Source: CAD feature listing. Evaluate the final solid. Frame: model axes, mm. Face numbers are marked on the shaded views. A direction names the side the tool comes from. Give positions to 0.01 mm unless a question says otherwise; leave off trailing zeros. Order: outer loops, then holes, each group sorted by start corner. A loop starts at its lowest first (then second) coordinate and runs counter-clockwise, first axis right, second up. Notation, with made-up numbers: M 70,80 L 81,80 A29 cw 81,117 Z; hole C 57.25,1 d8. An arc over 180 degrees is marked long. Return JSON: item names as keys, results as strings.
Autodesk Inventor part; units mm, degrees
ref_plane "YZ Plane" through (0, 0, 0) normal (1, 0, 0) x (0, 1, 0)
ref_plane "XZ Plane" through (0, 0, 0) normal (0, 1, 0) x (-1, 0, 0)
ref_plane "XY Plane" through (0, 0, 0) normal (0, 0, 1) x (1, 0, 0)
sketch "スケッチ1" plane through (0, 0, 0) normal (0, 1, 0) x (-1, 0, 0)
  circle A0 centre (0, 0) radius 1.15
  circle A1 centre (0, 0) radius 2
  circle A2 centre (0, 0) radius 3
  line L0 (0, 0) -> (0, 3)
  line L1 (-2, 0) -> (2, 0)
  line L2 (2, 0) -> (2, -3)
  line L3 (2, -3) -> (-2, -3)
  line L4 (-2, -3) -> (-2, 0)
  line L5 (0, 0) -> (3, 0)
  line L6 (3, 0) -> (3, 3)
  line L7 (3, 3) -> (0, 3)
  line L8 (0, 3) -> (0, 0)
  point P0 (-2, -2.2361)
  point P1 (0, 2)
  point P2 (2, -2.2361)
  dimension "d1" = 4
  dimension "d2" = 6
  dimension "d0" = 2.3
extrude "押し出し1" add sketch "スケッチ1" along normal blind 3.2 contours A1 L4 A2 L0
extrude "押し出し2" add sketch "スケッチ1" along normal blind 4.5 contours L5 A2 L2 | A1 L0 A2 L5 | A2 L7 L6
extrude "押し出し3" add sketch "スケッチ1" against normal blind 1 contours L1 A1 A0 | A0 L0 A1 L1 | A0 L1 A1 L0 | L2 A2 L4 A1 | L5 A2 L2 | A1 L0 A2 L5 | A1 L4 A2 L0 | A2 L7 L6
sketch "スケッチ2" plane through (0, 4.5, 0) normal (0, 1, 0) x (1, 0, 0)
  circle A0 centre (0, 0) radius 1.15
  circle A1 centre (0, 0) radius 2
  circle A2 centre (0, 0) radius 3
  line L0 (0, 0) -> (-3, 0)
  line L1 (-3, 0) -> (-3, -3)
  line L2 (-3, -3) -> (0, -3)
  line L3 (0, -3) -> (0, 0)
  dimension "d9" = 2.3
  dimension "d10" = 4
  dimension "d11" = 6
extrude "押し出し4" add sketch "スケッチ2" along normal blind 1 contours A0 L0 A1 L3 | A0 L3 A1 L0 | L0 A2 L3 A1 | A1 L3 A2 L0 | A2 L2 L1
sketch "スケッチ3" plane through (-3, -1, 3) normal (0, 0, 1) x (1, 0, 0)
  line L0 (0, 6.5) -> (0, 0)
  line L1 (3, 5.5) -> (3, 6.5)
  line L2 (0, 0) -> (3, 0)
  line L3 (3, 0) -> (3, 6.5)
  line L4 (3, 6.5) -> (0, 6.5)
  line L5 (0, 6.5) -> (0, 0)
  point P0 (3, 1)
extrude "押し出し5" add sketch "スケッチ3" along normal blind 7
sketch "スケッチ4" plane through (-3, -1, 10) normal (0, 0, 1) x (1, 0, 0)
  line L0 (4.15, 0) -> (1.85, 0)
  line L1 (3, 0) -> (1.5, 0)
  line L2 (1.5, 0) -> (1.5, 1.5)
  line L3 (1.5, 1.5) -> (3, 1.5)
  line L4 (3, 1.5) -> (3, 0)
  point P0 (3, 1)
  dimension "d16" = 1.5
  dimension "d17" = 1.5
hole "穴1" at (-1.5, 0.5, 10) direction (0, 0, -1) diameter 1 end through all
sketch "スケッチ5" plane through (0, 3.2, 3) normal (1, 0, 0) x (0, 0, -1)
  point P0 (3, -3.2)
sketch "スケッチ7" plane through (0, 5.5, 0) normal (0, 1, 0) x (1, 0, 0)
  line L0 (0, -3) -> (0, -10)
  line L1 (0, -10) -> (-3, -10)
  line L2 (-3, -10) -> (-3, -50)
  line L3 (-3, -50) -> (0, -50)
  line L4 (0, -50) -> (0, -10)
  point P0 (0, 0)
  dimension "d33" = 3
  dimension "d34" = 40
sketch "スケッチ8" plane through (-3, -1, 10) normal (0, 0, 1) x (1, 0, 0)
  line L0 (0, 0) -> (0, 6.5)
  line L1 (0, 6.5) -> (4, 6.5)
  line L2 (4, 6.5) -> (4, 2.5)
  line L3 (4, 2.5) -> (0, 2.5)
  line L4 (0, 2.5) -> (0, 6.5)
  point P0 (3, 1)
  dimension "d35" = 4
  dimension "d36" = 4
extrude "押し出し7" add sketch "スケッチ8" along normal mid plane 8
sketch "スケッチ9" plane through (-3, -1, 14) normal (0, 0, 1) x (1, 0, 0)
  line L0 (0, 0) -> (0, 6.5)
  line L1 (0, 6.5) -> (2, 6.5)
  line L2 (2, 6.5) -> (2, 4.5)
  line L3 (2, 4.5) -> (0, 4.5)
  line L4 (0, 4.5) -> (0, 6.5)
  point P0 (3, 1)
  dimension "d39" = 2
  dimension "d40" = 2
hole "穴2" at (-1, 3.5, 14) direction (0, 0, -1) diameter 2 depth 3 tip angle 118
fillet "フィレット1" radius 2 1 edges at (1, 3.5, 6)
properties part number "srod1.2"
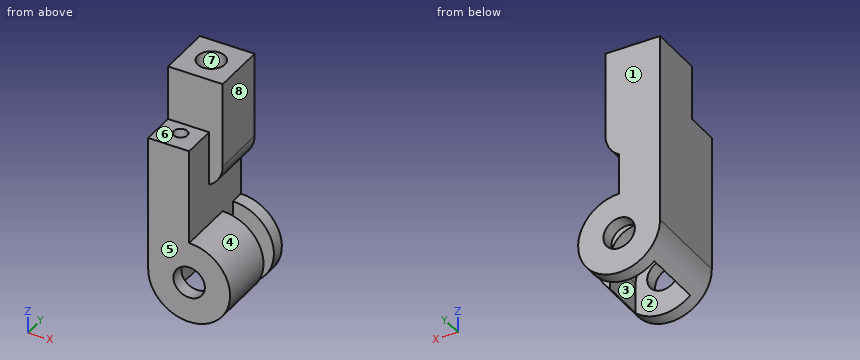
1. First-contact query: pin 1 (3 mm diameter, centred on x = 0, z = 0, fed in from +Y); pin 2 (2 mm diameter, centred on y = 0, z = 5, fed in from +X); pin 3 (1 mm diameter, centred on x = 2.5, z = 4, fed in from +Y); pin 4 (3 mm diameter, centred on y = 4, z = 11.5, fed in from +X). Flat tips, straight axial feed; report the tip coordinate or a pass-through.
Evaluation:
{"pin 1": "stops at y = 5.5", "pin 2": "stops at x = 0", "pin 3": "passes through", "pin 4": "stops at x = 1"}
2. Ray query, probe 1 along X at (y, z) = (0.5, 3.5); probe 2 along Y at (x, z) = (-0.85, 1); probe 3 along Y at (x, z) = (-1, 12.4). Return the intervals inside material, ascending.
Evaluation:
{"probe 1": "x = -3 to -2, -1 to 0", "probe 2": "y = -1 to 0, 4.5 to 5.5", "probe 3": "y = 1.5 to 2.5, 4.5 to 5.5"}
3. Section query C-C (z = 0.5). Return loops of the section in (x, y).
Evaluation:
{"outline": "M -3,-1 L -1.04,-1 L -1.04,0 L -1.94,0 L -1.94,0.26 A0.5 cw -1.94,0.74 L -1.94,4.5 L -1.04,4.5 L -1.04,5.5 L -3,5.5 Z; M 1.04,-1 L 2.96,-1 L 2.96,3.2 L 1.94,3.2 L 1.94,0 L 1.04,0 Z; M 1.04,4.5 L 2.96,4.5 L 2.96,5.5 L 1.04,5.5 Z"}
4. Section query D-D (x = -0.7). State how many separate pieces and enclosed holes the cut face has, then the cut area to 3 significant figures.
Evaluation:
{"separate pieces": "3", "enclosed holes": "0", "area": "68.6 mm^2"}
5. Section query A-A (z = 12). Return loops of the section in (x, y).
Evaluation:
{"outline": "M -3,1.5 L 1,1.5 L 1,5.5 L -3,5.5 Z; hole C -1,3.5 d2"}
6. Set-up query: the marked faces 5, 6, 7 and 8. Return all of +Z, -Z, +X, -X, +Y, -Y with unobstructed straight access to the full face (end or side cutting, diameter ignored); none if empty.
Evaluation:
{"face 5": "+Z, -Z, +X, -X, -Y", "face 6": "+Z, +X, -X, -Y", "face 7": "+Z", "face 8": "+Z, +X, +Y, -Y"}
7. Section query B-B (y = -0.5). Return loops of the section in (x, z).
Evaluation:
{"outline": "M -3,0 A3 ccw long 0,3 L 0,10 L -3,10 Z; hole C 0,0 d2.3"}
8. Draft query along X for the marked faces 1, 2, 3 and 4. Return one class per face: pulls with the +X half, pulls with the -X half, needs draft (parallel to the pull), parting line crosses it, or undercut.
Evaluation:
{"face 1": "needs draft", "face 2": "undercut", "face 3": "undercut", "face 4": "parting line crosses it"}
